Could you check a few things on this model? Use its own coordinates, in mm. A direction names the side the tool comes from. Coordinates: 2 decimals unless noted, no trailing zeros. Loops run counter-clockwise (first coordinate to the right, second up) from the corner with the lowest first, then second, coordinate; pieces in that order, holes last.
1) Imagine slicing it at D-D on x = -14. Please give me the cut outline in (y, z), plus the area to 3 significant figures.
2) Imagine slicing it at C-C on z = 2.5. Give the number of separate pieces and of enclosed holes in the cut face, plus the area to 3 significant figures.
3) Will these pins go through, and if not, where does the flat tip stop? P1, Ø1, axis at x = -1, z = 10.5, coming from the +Y side (3 decimals); P2, Ø6.5, axis at y = -11.5, z = 11.5, coming from the +X side; P3, Ø1.5, axis at y = 31, z = 5, coming from the -X side; P4, Ø1, axis at x = -13, y = 18.5, coming from the +Z side.
4) Imagine slicing it at B-B on z = 14.75. Please give me the cut outline in (x, y) (1 decimal).
5) Imagine slicing it at A-A on x = 0. Please give me the cut outline in (y, z) (3 decimals), plus the area to 3 significant figures.
6) Thinking about a two-plate mould opening in X: for faces 5 (the face through (-10, 0, 19.05)), 6 (the face through (12.7, 0, 13)), 7 (the face through (0.215, 30.787, 3.131)), which applies, released by +X, released by -X, zero draft, split by the parting line, or undercut?
7) For faces 1 (the face through (0.03, 23.83, 7.62)), 2 (the face through (2, 22.225, 13)), 3 (the face through (0, -25.4, 13)), 4 (the face through (3, 25.4, 13)), which set-ups out of +Z, -Z, +X, -X, +Y, -Y let a thin tool reach every point of the face, with its end or its side?
8) If I drill on line 1 along X through (y, z) = (2.5, 10.25) (3 decimals); line 2 along Y through (x, z) = (8, 13.75) (3 decimals); line 3 along Y through (x, z) = (-10.5, 10.5), over which ranges is the centre line in solid material (lowest first)?
```python
from build123d import *

# Parameters (mm, degrees)
F0_R     = 0.628762
F1_DEPTH = 6.35
F2_W     = 25.4
F2_H     = 50.8
F2_W_2   = 19.05
F2_H_2   = 44.45
F3_DEPTH = 12.7
F5_DEPTH = 25.4


with BuildPart() as f1:
    # F0 (on Top) → F1 (new body)
    with BuildSketch(Plane.XY):
        with BuildLine():
            ThreePointArc((12.7, 38.1), (0, 30.785806), (-12.7, 38.1))
            ThreePointArc((-12.7, 38.1), (-28.751062, 50.349914), (-36.331557, 31.635399))
            ThreePointArc((-36.331557, 31.635399), (-23.370243, 1.385669), (-34.742058, -29.496748))
            ThreePointArc((-34.742058, -29.496748), (-34.825441, -29.589354), (-34.909084, -29.681727))
            ThreePointArc((-34.909084, -29.681727), (-29.901368, -49.975508), (-12.7, -38.1))
            ThreePointArc((-12.7, -38.1), (0, -30.785806), (12.7, -38.1))
            ThreePointArc((12.7, -38.1), (29.901368, -49.975508), (34.909084, -29.681727))
            ThreePointArc((34.909084, -29.681727), (34.825441, -29.589354), (34.742058, -29.496748))
            ThreePointArc((34.742058, -29.496748), (23.370243, 1.385669), (36.331557, 31.635399))
            ThreePointArc((36.331557, 31.635399), (28.751062, 50.349914), (12.7, 38.1))
        make_face()
        with Locations((-24.636335, -44.956376)):
            Circle(F0_R, mode=Mode.SUBTRACT)
        with Locations((-32.256376, -37.336335)):
            Circle(F0_R, mode=Mode.SUBTRACT)
        with Locations((-26.163665, -31.243624)):
            Circle(F0_R, mode=Mode.SUBTRACT)
        with Locations((-18.543624, -38.863665)):
            Circle(F0_R, mode=Mode.SUBTRACT)
        with Locations((18.543624, -38.863665)):
            Circle(F0_R, mode=Mode.SUBTRACT)
        with Locations((24.636335, -44.956376)):
            Circle(F0_R, mode=Mode.SUBTRACT)
        with Locations((26.163665, -31.243624)):
            Circle(F0_R, mode=Mode.SUBTRACT)
        with Locations((32.256376, -37.336335)):
            Circle(F0_R, mode=Mode.SUBTRACT)
        with Locations((-32.256376, 37.336335)):
            Circle(F0_R, mode=Mode.SUBTRACT)
        with Locations((-26.163665, 31.243624)):
            Circle(F0_R, mode=Mode.SUBTRACT)
        with Locations((-24.636335, 44.956376)):
            Circle(F0_R, mode=Mode.SUBTRACT)
        with Locations((-18.543624, 38.863665)):
            Circle(F0_R, mode=Mode.SUBTRACT)
        with Locations((18.543624, 38.863665)):
            Circle(F0_R, mode=Mode.SUBTRACT)
        with Locations((26.163665, 31.243624)):
            Circle(F0_R, mode=Mode.SUBTRACT)
        with Locations((32.256376, 37.336335)):
            Circle(F0_R, mode=Mode.SUBTRACT)
        with Locations((24.636335, 44.956376)):
            Circle(F0_R, mode=Mode.SUBTRACT)
        with BuildLine():
            ThreePointArc((-34.909084, -29.681727), (-34.825441, -29.589354), (-34.742058, -29.496748))
            ThreePointArc((-34.742058, -29.496748), (-34.826025, -29.588828), (-34.909084, -29.681727))
        make_face()
        with BuildLine():
            ThreePointArc((34.909084, -29.681727), (34.826025, -29.588828), (34.742058, -29.496748))
            ThreePointArc((34.742058, -29.496748), (34.825441, -29.589354), (34.909084, -29.681727))
        make_face()
    extrude(amount=F1_DEPTH)

    # F2 (on face) → F3 (join)
    with BuildSketch(Plane.XY.offset(6.35)):
        Rectangle(F2_W, F2_H)
        Rectangle(F2_W_2, F2_H_2, mode=Mode.SUBTRACT)
    extrude(amount=F3_DEPTH)

    # F4 (on face) → F5 (cut)
    with BuildSketch(Plane(origin=(0, 25.4, 0), x_dir=(-1, 0, 0), z_dir=(0, 1, 0))):
        with BuildLine():
            Line((1.5875, 19.05), (-1.5875, 19.05))
            Line((-1.5875, 19.05), (-1.5875, 9.2075))
            ThreePointArc((-1.5875, 9.2075), (0, 7.62), (1.5875, 9.2075))
            Line((1.5875, 9.2075), (1.5875, 19.05))
        make_face()
    extrude(amount=-F5_DEPTH, mode=Mode.SUBTRACT)


solid = f1.part
```
Filled in:
1. outline: (-43.7, 0) - (43.7, 0) - (43.7, 6.35) - (-43.7, 6.35) - close
1. area: 555 mm2
2. separate pieces: 1
2. enclosed holes: 16
2. area: 5,170 mm2
3. P1: stops at y = -22.225
3. P2: stops at x = 12.7
3. P3: stops at x = -36.4
3. P4: stops at z = 19.05
4. outline: (-12.7, -25.4) - (12.7, -25.4) - (12.7, 25.4) - (1.6, 25.4) - (1.6, 22.2) - (9.5, 22.2) - (9.5, -22.2) - (-9.5, -22.2) - (-9.5, 22.2) - (-1.6, 22.2) - (-1.6, 25.4) - (-12.7, 25.4) - close
5. outline: (-30.786, 0) - (30.786, 0) - (30.786, 6.35) - (25.4, 6.35) - (25.4, 7.62) - (22.225, 7.62) - (22.225, 6.35) - (-22.225, 6.35) - (-22.225, 19.05) - (-25.4, 19.05) - (-25.4, 6.35) - (-30.786, 6.35) - close
5. area: 435 mm2
6. face 5: zero draft
6. face 6: released by +X
6. face 7: undercut
7. face 1: +Z, +Y
7. face 2: +Z
7. face 3: +Z, +X, -X, -Y
7. face 4: +Z, +X, -X, +Y
8. line 1: x = -12.7 to -9.525, 9.525 to 12.7
8. line 2: y = -25.4 to -22.225, 22.225 to 25.4
8. line 3: y = -25.4 to 25.4
